```python
from build123d import *

# Parameters (mm, degrees)
ESQUISSE1_R             = 9
BOSS_EXTRU_1_DEPTH      = 7
ESQUISSE2_W             = 5.8
ESQUISSE2_H             = 2.4
ENL_V_MAT_EXTRU_1_DEPTH = 15.525839046
ESQUISSE7_R             = 2.95
ENL_V_MAT_EXTRU_8_DEPTH = 21.802884576
CHANFREIN1_SIZE         = 2.5
CHANFREIN1_SIZE_2       = 2.457485256
ESQUISSE9_R             = 3.95
BOSS_EXTRU_2_DEPTH      = 7
ENL_V_MAT_EXTRU_9_DEPTH = 19.92088803


# Read off the part's stored shape, not the designer's step: Enlèv. mat.-Extru.2
with BuildPart() as part:
    # Esquisse1 → Boss.-Extru.1 (new body)
    with BuildSketch(Plane.XY):
        Circle(ESQUISSE1_R)
    extrude(amount=BOSS_EXTRU_1_DEPTH)

    # Esquisse2 → Enlèv. mat.-Extru.1 (cut, through all)
    with BuildSketch(Plane(origin=(0, 0, 0), x_dir=(-1, 0, 0), z_dir=(0, 0, -1))):
        with Locations((0, 4.2)):
            Rectangle(ESQUISSE2_W, ESQUISSE2_H)
    extrude(amount=-ENL_V_MAT_EXTRU_1_DEPTH, mode=Mode.SUBTRACT)

    # Enlèv. mat.-Extru.2 outline → Enlèv. mat.-Extru.2 (revolve, cut)
    with BuildSketch(Plane.XY.offset(3.5)):
        Polygon((0, 5.4), (1.558107844, 5.4), (1.49526864, 9.000055608), (0, 9.000055608), align=None)
        Polygon((1.6, 3), (0, 3), (0, 1), (1.56508987, 1), align=None)
    revolve(axis=Axis((0, 0, 3.5), (0, 1, 0)), mode=Mode.SUBTRACT)

    # Esquisse7 → Enlèv. mat.-Extru.8 (cut, through all)
    with BuildSketch(Plane(origin=(0, 8.4, 0), x_dir=(1, 0, 0), z_dir=(0, 1, 0))):
        with Locations(Location((0, -3.5, 0), (0, 0, 90))):
            Circle(ESQUISSE7_R)
    extrude(amount=ENL_V_MAT_EXTRU_8_DEPTH, mode=Mode.SUBTRACT)

    # Chanfrein1
    # the kernel refuses this chamfer: 2.5, 2.457485256 mm, written as the material it takes off along each edge
    with BuildSketch(Plane(origin=(0, 8.4, 3.5), x_dir=(1, 0, 0), z_dir=(0, 0, 1))) as chanfrein1_piece_1_section:
        Polygon((1.50574265 + CHANFREIN1_SIZE, 0), (1.50574265 + CHANFREIN1_SIZE_2 * 0.0174524063286, -CHANFREIN1_SIZE_2 * 0.999847695023), (1.50574265, 0), align=None)
    chanfrein1_piece_1 = revolve(axis=Axis((0, 8.4, 3.5), (0, 1, 0)), mode=Mode.PRIVATE)
    chanfrein1_piece_1 = chanfrein1_piece_1 & Plane(origin=(0, 6.666447792, 3.5), x_dir=(0, 0, -1), z_dir=(0, -1, 0)) * Cylinder(2.95, 17, mode=Mode.PRIVATE)
    add(chanfrein1_piece_1, mode=Mode.SUBTRACT)

    # Esquisse9 → Boss.-Extru.2 (add)
    with BuildSketch(Plane.XY.offset(7)):
        with Locations((0, -1)):
            Circle(ESQUISSE9_R)
    extrude(amount=BOSS_EXTRU_2_DEPTH)

    # Esquisse10 → Enlèv. mat.-Extru.9 (cut, through all)
    with BuildSketch(Plane(origin=(0, 0, 0), x_dir=(-1, 0, 0), z_dir=(0, 0, -1))):
        with BuildLine():
            Line((-1.532970972, 2.1), (1.532970972, 2.1))
            ThreePointArc((1.532970972, 2.1), (0, -2.6), (-1.532970972, 2.1))
        make_face()
    extrude(amount=-ENL_V_MAT_EXTRU_9_DEPTH, mode=Mode.SUBTRACT)


solid = part.part
```
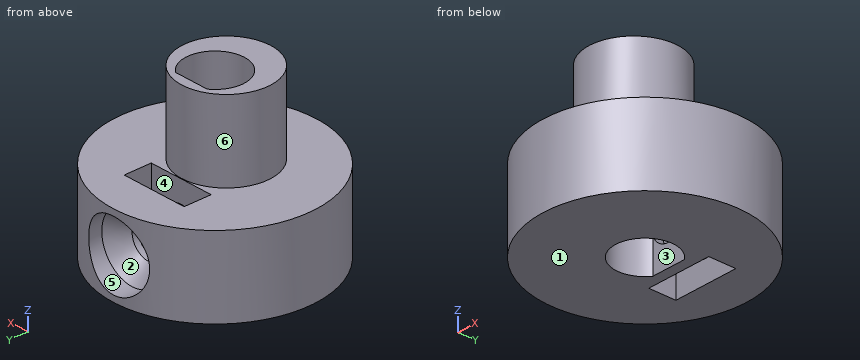
Here's how the part is built. I have some questions about the finished solid (model axes, mm). Face numbers are marked on the shaded views. A direction names the side the tool comes from. Round coordinates to 2 decimals unless told otherwise and drop trailing zeros. Write each loop counter-clockwise with the first axis right and the second up, starting at its lowest first coordinate (ties: lowest second). Pieces come first, ordered by that corner, then holes. Notation, with made-up numbers: M 76,-19.75 L 94,-19.75 A24 cw 94,-4.75 Z; hole C -35.5,37 d8. An arc over 180 degrees is marked long. Answer as CSV lines item,"result". Start each with the question number.
1. Suppose I cut it at D-D on x = 0. Count the separate pieces of the cut face and the enclosed holes in it, then the cut area to 3 significant figures.
2. Thinking about a two-plate mould opening in Y: for the marked faces 1, 2 and 3, which applies, released by +Y, released by -Y, zero draft, split by the parting line, or undercut?
3. I need wall thicknesses on probe 1 along Y at (x, z) = (0, 1.75); probe 2 along Z at (x, y) = (0, 8.45); probe 3 along Z at (x, y) = (-3.25, -8). Which ranges of each line are inside material? Lowest first, please.
4. Suppose I cut it at B-B on z = 12.75. Write out the boundary of the cut face in (x, y).
5. Suppose I cut it at C-C on y = 7.75. Write out the boundary of the cut face in (x, z), then the cut area to 3 significant figures.
6. On a 3-axis mill with a long thin cutter (end or side, diameter ignored), from which of +Z, -Z, +X, -X, +Y, -Y can I reach the whole of each face in a straight line? I mean the marked faces 4, 5 and 6. Say none if no direction works.
7. I'm going to push flat-ended pins straight in: pin 1 Ø1.5 at (y, z) = (-3.5, 2.5) entering from -X; pin 2 Ø5 at (y, z) = (6, 4) entering from -X; pin 3 Ø3 at (x, z) = (0, 4.5) entering from +Y. Where does each tip first touch, or does it pass through?
8. Suppose I cut it at A-A on y = 3.75. Write out the boundary of the cut face in (x, z).
Check result:
1,separate pieces,"5"
1,enclosed holes,"0"
1,area,"78.1 mm2"
2,face 1,"zero draft"
2,face 2,"released by +Y"
2,face 3,"undercut"
3,probe 1,"y = -9 to -2.6, 2.1 to 3, 5.4 to 6.14"
3,probe 2,"z = 0 to 0.55, 6.45 to 7"
3,probe 3,"z = 0 to 7"
4,outline,"C 0,-1 d7.9; hole M -1.53,2.1 A2.6 ccw long 1.53,2.1 Z"
5,outline,"M -4.58,0 L 4.58,0 L 4.58,7 L -4.58,7 Z; hole C 0,3.5 d5.9"
5,area,"36.7 mm2"
6,face 4,"+Z, -Z"
6,face 5,"+Y"
6,face 6,"+Z"
7,pin 1,"stops at x = -8.57"
7,pin 2,"stops at x = -8.29"
7,pin 3,"stops at y = 6.89"
8,outline,"M -8.18,0 L -2.9,0 L -2.9,7 L -8.18,7 Z; M 2.9,0 L 8.18,0 L 8.18,7 L 2.9,7 Z"
